Verification items for the finished model (mm, model axes). A direction names the side the tool comes from. Coordinates: 2 decimals unless noted, no trailing zeros. Order: outer loops, then holes, each group sorted by start corner. A loop starts at its lowest first (then second) coordinate and runs counter-clockwise, first axis right, second up. Notation, with made-up numbers: (19.25, -25) -> (39.25, -25) arc R7 ccw to (39.25, -18) -> close; hole circle Ø9 at (30, 6.25). An arc over 180 degrees is marked (long way). Answer as CSV lines item,"result".
```python
from build123d import *

# Parameters (mm, degrees)
SKETCH1_R           = 5
SKETCH1_R_2         = 3
BOSS_EXTRUDE1_DEPTH = 15
SKETCH2_R           = 5
SKETCH2_R_2         = 3
BOSS_EXTRUDE2_DEPTH = 15
FILLET1_R           = 2
SKETCH3_W           = 7.3092156
SKETCH3_H           = 4.6
CUT_EXTRUDE1_DEPTH  = 15
FILLET2_R           = 1
SKETCH4_W           = 6.886340675
SKETCH4_H           = 4.4
CUT_EXTRUDE2_DEPTH  = 15
FILLET3_R           = 0.5


with BuildPart() as part:
    # Sketch1 → Boss-Extrude1 (new body)
    with BuildSketch(Plane(origin=(0, 0, 0), x_dir=(1, 0, 0), z_dir=(0, 1, 0))):
        Circle(SKETCH1_R)
        Circle(SKETCH1_R_2, mode=Mode.SUBTRACT)
    extrude(amount=BOSS_EXTRUDE1_DEPTH)

    # Sketch2 → Boss-Extrude2 (add)
    with BuildSketch(Plane(origin=(0, 15, 0), x_dir=(1, 0, 0), z_dir=(0, 1, 0))):
        with Locations((8.100044145, -0.002335254)):
            Circle(SKETCH2_R)
        with Locations((8.100044145, -0.002335254)):
            Circle(SKETCH2_R_2, mode=Mode.SUBTRACT)
    extrude(amount=-BOSS_EXTRUDE2_DEPTH)

    # Fillet1
    fillet1_edges = [part.edges().sort_by_distance(p)[0] for p in [
        (4.050867406, 7.5, -2.930950913),
        (4.049176739, 7.5, 2.933286167),
    ]]
    fillet(fillet1_edges, radius=FILLET1_R)

    # Sketch3 → Cut-Extrude1 (cut)
    with BuildSketch(Plane.XZ):
        with Locations((-3.6546078, 0)):
            Rectangle(SKETCH3_W, SKETCH3_H)
    extrude(amount=-CUT_EXTRUDE1_DEPTH, mode=Mode.SUBTRACT)

    # Fillet2
    fillet2_edges = [part.edges().sort_by_distance(p)[0] for p in [
        (-4.439594576, 7.5, 2.3),
        (-4.439594576, 7.5, -2.3),
    ]]
    fillet(fillet2_edges, radius=FILLET2_R)

    # Sketch4 → Cut-Extrude2 (cut)
    with BuildSketch(Plane(origin=(0, 15, 0), x_dir=(1, 0, 0), z_dir=(0, 1, 0))):
        with Locations((11.966816287, -0.002335254)):
            Rectangle(SKETCH4_W, SKETCH4_H)
    extrude(amount=-CUT_EXTRUDE2_DEPTH, mode=Mode.SUBTRACT)

    # Fillet3
    fillet3_edges = [part.edges().sort_by_distance(p)[0] for p in [
        (12.590033009, 7.5, -2.197664746),
        (12.590033009, 7.5, 2.202335254),
    ]]
    fillet(fillet3_edges, radius=FILLET3_R)


solid = part.part
```
Item 1: Section check C-C, the plane z = 0. Record the boundary of the cut face in (x, y), plus the area to 3 significant figures.
Answer list:
outline,"(3, 0) -> (5.1, 0) -> (5.1, 15) -> (3, 15) -> close"
area,"31.5 mm2"
Item 2: Thickness scan on line 1 (Z direction, x = 0, y = 7); line 2 (X direction, y = 11.75, z = 0); line 3 (Z direction, x = 9.25, y = 5.5). Record the ranges inside material, lowest first.
Answer list:
line 1,"-5 to -3, 3 to 5"
line 2,"3 to 5.1"
line 3,"-4.86 to -2.77, 2.77 to 4.87"
Item 3: Release check for a two-part mould opening along Z. For faces 3 (the cylindrical face through (3, 7, 0)), 4 (the cylindrical face through (8.93, 7.61, -4.93)), 5 (the cylindrical face through (5.1, 7.6, -0.1)), 6 (the cylindrical face through (0, 7, 5)) record: +Z half, -Z half, draft (parallel to the pull), parting line (faces both ways), or undercut.
Answer list:
face 3,"undercut"
face 4,"-Z half"
face 5,"undercut"
face 6,"+Z half"
Item 4: Tool access check on faces 1 (the cylindrical face through (0, 7, -5)), 2 (the flat face through (11, 8, 2.202)). Record the directions out of +Z, -Z, +X, -X, +Y, -Y that give a thin tool (end or side, any length) a straight path to the whole face; none if there is none.
Answer list:
face 1,"-Z, +Y, -Y"
face 2,"+X, +Y, -Y"
Item 5: Depth check by flat-ended pin: pin 1 Ø3 at (x, y) = (6, 11.5) entering from +Z; pin 2 Ø1 at (x, y) = (-0.5, 6.5) entering from -Z; pin 3 Ø3.5 at (x, z) = (8.1, 0) entering from -Y; pin 4 Ø1 at (x, y) = (3.5, 8) entering from -Z. Enter the tip coordinate at first touch or a pass-through.
Answer list:
pin 1,"z = 4.97"
pin 2,"z = -5"
pin 3,"through"
pin 4,"z = -4.01"
Item 6: Section check B-B, the plane x = 8.75. Record the boundary of the cut face in (y, z), plus the area to 3 significant figures.
Answer list:
outline,"(0, -4.96) -> (15, -4.96) -> (15, -2.93) -> (0, -2.93) -> close; (0, 2.93) -> (15, 2.93) -> (15, 4.96) -> (0, 4.96) -> close"
area,"60.9 mm2"
Item 7: Section check A-A, the plane x = 0. Record the boundary of the cut face in (y, z).
Answer list:
outline,"(0, -5) -> (15, -5) -> (15, -3) -> (0, -3) -> close; (0, 3) -> (15, 3) -> (15, 5) -> (0, 5) -> close"
